The listing builds one solid part. Answer for the finished solid, in the listing's coordinates (mm). Round coordinates to 2 decimals unless told otherwise and drop trailing zeros. Order: outer loops, then holes, each group sorted by start corner. A loop starts at its lowest first (then second) coordinate and runs counter-clockwise, first axis right, second up. Notation, with made-up numbers: (33.25, -10.75) -> (92.25, -10.75) arc R33 ccw to (92.25, 22.25) -> close; hole circle Ø1 at (18, 36.5). An arc over 180 degrees is marked (long way). Return JSON: item names as keys, results as strings. Group by question number.
(1) The part is cut by section D-D (y = 22). Determine the outline of the cut face in (x, z), plus the area to 3 significant figures.
(2) Consider line 1 (Y direction, x = 1, z = 34.5); line 2 (Y direction, x = 4.75, z = 34); line 3 (Z direction, x = 9.75, y = 24.5). Determine where each line is inside the solid, lowest interval first. Write a range as [from, to].
(3) The part is cut by section C-C (x = 9). Determine the outline of the cut face in (y, z), plus the area to 3 significant figures.
(4) The part is cut by section A-A (y = 11.5). Determine the outline of the cut face in (x, z), plus the area to 3 significant figures.
(5) The part is cut by section B-B (z = 22.25). Determine the outline of the cut face in (x, y).
(6) Determine the mould class of faces 1 (the face through (6, -3, 15.689)), 2 (the face through (12.7, -22, 29)), 3 (the face through (6.3, 22.8, 37.2)) for opening direction Z: +Z half, -Z half, draft (parallel to the pull), parting line (faces both ways), or undercut.
Autodesk Inventor part; units mm, degrees
ref_plane "YZ Plane" through (0, 0, 0) normal (1, 0, 0) x (0, 1, 0)
ref_plane "XZ Plane" through (0, 0, 0) normal (0, 1, 0) x (-1, 0, 0)
ref_plane "XY Plane" through (0, 0, 0) normal (0, 0, 1) x (1, 0, 0)
sketch "Sketch1" plane through (0, 0, 0) normal (1, 0, 0) x (0, 1, 0)
  line L0 (35.5795, 41.0894) -> (-40.6205, 41.0894)
  line L1 (-40.6205, 41.0894) -> (-40.6205, 15.6894)
  line L2 (-40.6205, 15.6894) -> (35.5795, 15.6894)
  line L3 (35.5795, 15.6894) -> (35.5795, 41.0894)
  point P0 (0, 0)
  dimension "d0" = 76.2
  dimension "d1" = 25.4
extrude "Extrusion1" add sketch "Sketch1" along normal blind 12.7
sketch "Sketch2" plane through (12.7, 0, 0) normal (1, 0, 0) x (0, 0, -1)
  line L0 (-15.6894, -40.6205) -> (-15.6894, 35.5795)
  line L1 (-41.0894, 35.5795) -> (-41.0894, -40.6205)
  line L2 (-15.6894, 35.5795) -> (-41.0894, 35.5795)
  line L3 (-41.0894, -40.6205) -> (-15.6894, -40.6205)
  point P0 (0, 0)
  point P1 (-34.7394, 22.8795)
  point P2 (-22.0394, 22.8795)
  point P3 (-34.7394, -27.9205)
  point P4 (-22.0394, -27.9205)
  point P5 (-28.3894, -15.2205)
  point P6 (-28.3894, 10.1795)
  dimension "d4" = 0
  dimension "d5" = 0
  dimension "d6" = 6.35
  dimension "d7" = 6.35
  dimension "d8" = 12.7
  dimension "d9" = 25.4
  dimension "d10" = 12.7
  dimension "d11" = 25.4
  dimension "d12" = 12.7
  dimension "d13" = 6.35
  dimension "d14" = 6.35
  dimension "d15" = 12.7
hole "Hole1" at (12.7, 22.8795, 34.7394) at (12.7, 22.8795, 22.0394) at (12.7, -27.9205, 34.7394) at (12.7, -27.9205, 22.0394) at (12.7, -15.2205, 28.3894) at (12.7, 10.1795, 28.3894) direction (-1, 0, 0) diameter 4.9276 end through all
sketch "Sketch3" plane through (0, -40.6205, 41.0894) normal (0, 0, 1) x (1, 0, 0)
  arc A0 (12.7, 38.354) -> (12.7, 37.846) centre (12.7, 38.1) ccw
  line L0 (12.7, 76.2) -> (12.7, 0)
  line L1 (0, 76.2) -> (12.7, 76.2)
  point P0 (0, 40.6205)
  dimension "d23" = 0.254
  dimension "d24" = 38.1
  dimension "d27" = 0
extrude "Extrusion2" cut sketch "Sketch3" against normal blind 26.9875
properties part number "CabinetBraket"
Answer below:
{
 "1": {"outline": "(0, 15.69) -> (12.7, 15.69) -> (12.7, 19.74) -> (0, 19.74) -> close; (0, 24.34) -> (12.7, 24.34) -> (12.7, 32.44) -> (0, 32.44) -> close; (0, 37.04) -> (12.7, 37.04) -> (12.7, 41.09) -> (0, 41.09) -> close", "area": "206 mm²"},
 "2": {"line 1": "y = [-40.62, -30.37], [-25.47, 20.43], [25.33, 35.58]", "line 2": "y = [-40.62, -30.27], [-25.57, 20.53], [25.23, 35.58]", "line 3": "z = [15.69, 20.18], [23.9, 32.88], [36.6, 41.09]"},
 "3": {"outline": "(-40.62, 15.69) -> (35.58, 15.69) -> (35.58, 41.09) -> (-40.62, 41.09) -> close; hole circle Ø4.93 at (-27.92, 22.04); hole circle Ø4.93 at (-27.92, 34.74); hole circle Ø4.93 at (-15.22, 28.39); hole circle Ø4.93 at (10.18, 28.39); hole circle Ø4.93 at (22.88, 22.04); hole circle Ø4.93 at (22.88, 34.74)", "area": "1,820 mm²"},
 "4": {"outline": "(0, 15.69) -> (12.7, 15.69) -> (12.7, 26.31) -> (0, 26.31) -> close; (0, 30.47) -> (12.7, 30.47) -> (12.7, 41.09) -> (0, 41.09) -> close", "area": "270 mm²"},
 "5": {"outline": "(0, -40.62) -> (12.7, -40.62) -> (12.7, -30.38) -> (0, -30.38) -> close; (0, -25.47) -> (12.7, -25.47) -> (12.7, -2.77) arc R0.25 cw to (12.7, -2.27) -> (12.7, 20.42) -> (0, 20.42) -> close; (0, 25.33) -> (12.7, 25.33) -> (12.7, 35.58) -> (0, 35.58) -> close"},
 "6": {"face 1": "-Z half", "face 2": "draft", "face 3": "undercut"}
}
